Verification items for the finished model (mm, model axes). A direction names the side the tool comes from. Give positions to 0.01 mm unless a question says otherwise; leave off trailing zeros. Write each loop counter-clockwise with the first axis right and the second up, starting at its lowest first coordinate (ties: lowest second). Pieces come first, ordered by that corner, then holes. Notation, with made-up numbers: (68.25, 22) - (89.25, 22) arc R22 ccw to (89.25, 28) - close; hole circle Ø6 at (-35, 19). An arc over 180 degrees is marked (long way). Answer as a JSON object with one key per item and string values. Group by question number.
Item 1: Tool access check on faces 1 (the face through (0, 1.5, -2)), 2 (the face through (12, -6.35, -2)). Record the directions out of +Z, -Z, +X, -X, +Y, -Y that give a thin tool (end or side, any length) a straight path to the whole face; none if there is none.
Item 2: Sectioned sample at B-B, the plane z = -1.6. Record the boundary of the cut face in (x, y).
Item 3: Go/stop test with flat-tipped pins: pin 1 (3.5 mm diameter, centred on x = 25, y = 0, fed in from +Z); pin 2 (1 mm diameter, centred on y = -5, z = -2.5, fed in from +X). Record where each tip stops, or that it passes through.
Item 4: Draft check along X on faces 3 (the face through (-6.35, 0.14, -1.57)), 4 (the face through (13, 6.35, -2)), 5 (the face through (31.35, -0.14, -1.57)), 6 (the face through (0.07, -2.05, -1.57)). Enter one of: +X half, -X half, draft (parallel to the pull), parting line (faces both ways), or undercut.
Item 5: Scan lines: line 1 along Y through (x, z) = (25, -0.7); line 2 along X through (y, z) = (0.25, -2.7); line 3 along Y through (x, z) = (0, -0.75). Record each from-to range of solid material in increasing order. Write a range as [from, to].
Item 6: Sectioned sample at C-C, the plane x = 26. Record the boundary of the cut face in (y, z) (3 decimals).
Item 7: Sectioned sample at D-D, the plane x = 0.5. Record the boundary of the cut face in (y, z) (3 decimals), and give its area (3 significant figures).
Item 8: Sectioned sample at A-A, the plane y = 0. Record the boundary of the cut face in (x, z) (3 decimals), and give its area (3 significant figures).
```python
from build123d import *

# Parameters (mm, degrees)
SKETCH1_R      = 3
EXTRUDE1_DEPTH = 3.175


with BuildPart() as part:
    # Sketch1 → Extrude1 (new body)
    with BuildSketch(Plane.XY):
        with BuildLine():
            Line((25, 6.35), (0, 6.35))
            ThreePointArc((0, 6.35), (-6.35, 0), (0, -6.35))
            Line((0, -6.35), (25, -6.35))
            ThreePointArc((25, -6.35), (31.35, 0), (25, 6.35))
        make_face()
        with Locations((25, 0)):
            Circle(SKETCH1_R, mode=Mode.SUBTRACT)
        with BuildLine():
            Line((-1.397318861, 1.5), (1.397318861, 1.5))
            ThreePointArc((1.397318861, 1.5), (0, -2.05), (-1.397318861, 1.5))
        make_face(mode=Mode.SUBTRACT)
    extrude(amount=-EXTRUDE1_DEPTH)


solid = part.part
```
Geometry check:
{
 "1": {"face 1": "+Z, -Z", "face 2": "+Z, -Z, +X, -X, -Y"},
 "2": {"outline": "(0, -6.35) - (25, -6.35) arc R6.35 ccw to (25, 6.35) - (0, 6.35) arc R6.35 ccw to start; hole (-1.4, 1.5) arc R2.05 ccw (long way) to (1.4, 1.5) - close; hole circle Ø6 at (25, 0)"},
 "3": {"pin 1": "through", "pin 2": "x = 29.48"},
 "4": {"face 3": "-X half", "face 4": "draft", "face 5": "+X half", "face 6": "undercut"},
 "5": {"line 1": "[-6.35, -3], [3, 6.35]", "line 2": "[-6.35, -2.03], [2.03, 22.01], [27.99, 31.35]", "line 3": "[-6.35, -2.05], [1.5, 6.35]"},
 "6": {"outline": "(-6.271, -3.175) - (-2.828, -3.175) - (-2.828, 0) - (-6.271, 0) - close; (2.828, -3.175) - (6.271, -3.175) - (6.271, 0) - (2.828, 0) - close"},
 "7": {"outline": "(-6.35, -3.175) - (-1.988, -3.175) - (-1.988, 0) - (-6.35, 0) - close; (1.5, -3.175) - (6.35, -3.175) - (6.35, 0) - (1.5, 0) - close", "area": "29.2 mm^2"},
 "8": {"outline": "(-6.35, -3.175) - (-2.05, -3.175) - (-2.05, 0) - (-6.35, 0) - close; (2.05, -3.175) - (22, -3.175) - (22, 0) - (2.05, 0) - close; (28, -3.175) - (31.35, -3.175) - (31.35, 0) - (28, 0) - close", "area": "87.6 mm^2"}
}
